from build123d import *

# Parameters (mm, degrees)
EXTRU_MINCE1_DEPTH      = 40
ESQUISSE2_OUTSIDE_W     = 64.814
ESQUISSE2_OUTSIDE_H     = 54.814
ESQUISSE2_OUTSIDE_R     = 19.5
ESQUISSE2_OUTSIDE_R_2   = 16
ENL_V_MAT_EXTRU_1_DEPTH = 40


with BuildPart() as part:
    # Esquisse1 → Extru.-Mince1 (new body)
    with BuildSketch(Plane.XY):
        with BuildLine():
            ThreePointArc((0, 0), (5, 1), (10, 0))
            ThreePointArc((10, 0), (15, -1), (20, 0))
            ThreePointArc((20, 0), (25, 1), (30, 0))
            ThreePointArc((30, 0), (35, -1), (40, 0))
            ThreePointArc((40, 0), (45, 1), (50, 0))
            Line((50, 0), (49.884615385, -0.276923077))
            ThreePointArc((49.884615385, -0.276923077), (45, 0.7), (40.115384615, -0.276923077))
            ThreePointArc((40.115384615, -0.276923077), (35, -1.3), (29.884615385, -0.276923077))
            ThreePointArc((29.884615385, -0.276923077), (25, 0.7), (20.115384615, -0.276923077))
            ThreePointArc((20.115384615, -0.276923077), (15, -1.3), (9.884615385, -0.276923077))
            ThreePointArc((9.884615385, -0.276923077), (5, 0.7), (0.115384615, -0.276923077))
            Line((0.115384615, -0.276923077), (0, 0))
        make_face()
    extrude(amount=-EXTRU_MINCE1_DEPTH)

    # Esquisse2 outside → Enlèv. mat.-Extru.1 (cut)
    # profile 1 of 2: a face of its own
    with BuildSketch(Plane(origin=(0, 5, 0), x_dir=(-1, 0, 0), z_dir=(0, 1, 0))):
        with Locations((-25, -20)):
            Rectangle(ESQUISSE2_OUTSIDE_W, ESQUISSE2_OUTSIDE_H)
        with Locations(Location((-25.24411071, -19.869880187, 0), (0, 0, 103.767029359))):
            Circle(ESQUISSE2_OUTSIDE_R, mode=Mode.SUBTRACT)
    # profile 2 of 2: a face of its own
    with BuildSketch(Plane(origin=(0, 5, 0), x_dir=(-1, 0, 0), z_dir=(0, 1, 0))):
        with Locations(Location((-25.24411071, -19.869880187, 0), (0, 0, 106.859844414))):
            Circle(ESQUISSE2_OUTSIDE_R_2)
    extrude(amount=-ENL_V_MAT_EXTRU_1_DEPTH, mode=Mode.SUBTRACT)


solid = part.part
Build history of the part. All positions in model axes, mm. Coordinates: 2 decimals unless noted, no trailing zeros. Write each loop counter-clockwise with the first axis right and the second up, starting at its lowest first coordinate (ties: lowest second). Pieces come first, ordered by that corner, then holes.
(1) Cut at D-D on z = -10.5. List the corners of the cut face in (x, y) (3 decimals).
(2) Mould opens along X. For faces 1 (the cylindrical face through (35.413, -1.294, -6.452)), 2 (the cylindrical face through (41.901, 0.316, -19.693)), 3 (the cylindrical face through (8.343, 0.252, -19.702)), 4 (the cylindrical face through (25.1, 0.7, -2.5)) say: pulls with the +X half, pulls with the -X half, needs draft (parallel to the pull), parting line crosses it, or undercut.
(3) Cut at B-B on z = -21.5. List the corners of the cut face in (x, y), and give its area (3 significant figures).
(4) Drill centre lines: line 1 (Z direction, x = 31, y = -0.65); line 2 (Y direction, x = 42.5, z = -19); line 3 (Y direction, x = 41, z = -26). Where is each one in solid material? Low to high.
(5) Cut at C-C on z = -27. List the corners of the cut face in (x, y).
(6) Cut at A-A on x = 13. List the corners of the cut face in (y, z), and give its area (3 significant figures).
Working result:
1. outline: (8.143, 0.305) arc R12.7 cw to (9.885, -0.277) arc R13.3 ccw to (12.275, -1.018) - (12.275, -0.711) arc R13 cw to (10, 0) arc R13 ccw to (8.143, 0.614) - close; (38.214, -0.906) arc R13.3 ccw to (40.115, -0.277) arc R12.7 cw to (42.345, 0.419) - (42.345, 0.726) arc R13 ccw to (40, 0) arc R13 cw to (38.214, -0.597) - close
2. face 1: undercut
2. face 2: pulls with the +X half
2. face 3: pulls with the -X half
2. face 4: undercut
3. outline: (5.81, 0.67) arc R12.7 cw to (9.33, -0.06) - (9.33, 0.26) arc R13 ccw to (5.81, 0.97) - close; (41.16, 0.11) arc R12.7 cw to (44.68, 0.7) - (44.68, 1) arc R13 ccw to (41.16, 0.42) - close
3. area: 2.15 mm2
4. line 1: z = -38.5 to -34.8, -4.94 to -1.24
4. line 2: y = 0.45 to 0.76
4. line 3: y = 0.05 to 0.37
5. outline: (7.09, 0.53) arc R12.7 cw to (9.88, -0.28) arc R13.3 ccw to (10.92, -0.66) - (10.92, -0.34) arc R13 cw to (10, 0) arc R13 ccw to (7.09, 0.83) - close; (39.57, -0.49) arc R13.3 ccw to (40.12, -0.28) arc R12.7 cw to (43.39, 0.6) - (43.39, 0.9) arc R13 ccw to (40, 0) arc R13 cw to (39.57, -0.17) - close
6. outline: (-1.15, -35.05) - (-0.85, -35.05) - (-0.85, -30.17) - (-1.15, -30.17) - close; (-1.15, -9.57) - (-0.85, -9.57) - (-0.85, -4.69) - (-1.15, -4.69) - close
6. area: 2.96 mm2
